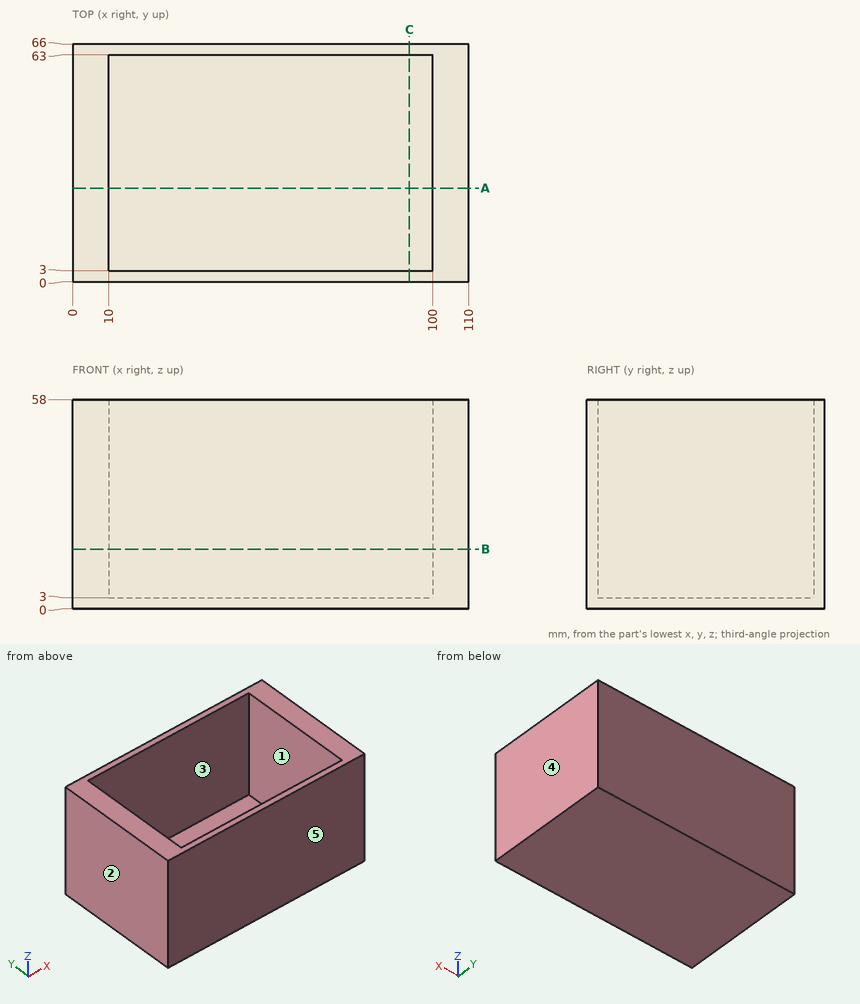
Part print with two shaded views. Sizes in mm from the minimum x, y, z corner. A direction names the side the tool comes from. Coordinates: 2 decimals unless noted, no trailing zeros. Write each loop counter-clockwise with the first axis right and the second up, starting at its lowest first coordinate (ties: lowest second). Pieces come first, ordered by that corner, then holes. Notation, with made-up numbers: (61, 62) -> (105, 62) arc R11 cw to (105, 69) -> close; hole circle Ø10 at (52.25, 76.25). An arc over 180 degrees is marked (long way). Return JSON: item names as keys, results as strings. Group by question number.
Q1. Cut at B-B, the plane z = 16.5. Give the cut face in (x, y).
Q2. Drill centre lines: line 1 (Y direction, x = 73, z = 9.5); line 2 (X direction, y = 10.5, z = 44); line 3 (Z direction, x = 31, y = 33.5). Where is each one in solid material? Low to high.
Q3. Which spindle directions (+Z, -Z, +X, -X, +Y, -Y) get a long thin tool onto all of the face, cutting with end or side? Do the marked faces 1 and 2. Say none if no direction does.
Q4. Pull direction Y, two halves, no side cores. Call the marked faces 3, 4 and 5: released by +Y, released by -Y, zero draft, split by the parting line, or undercut.
Q5. Cut at A-A, the plane y = 26. Give the cut face in (x, z).
Q6. Cut at C-C, the plane x = 93.5. Give the cut face in (y, z).
Q7. Flat gauge pins, fed straight in: pin 1 (6 mm diameter, centred on x = 92.5, y = 31, fed in from -Z); pin 2 (4 mm diameter, centred on x = 89.5, y = 57.5, fed in from +Z). Where does each tip first touch, or does it go through?
Returned:
{
 "1": {"outline": "(0, 0) -> (110, 0) -> (110, 66) -> (0, 66) -> close; hole (10, 3) -> (100, 3) -> (100, 63) -> (10, 63) -> close"},
 "2": {"line 1": "y = 0 to 3, 63 to 66", "line 2": "x = 0 to 10, 100 to 110", "line 3": "z = 0 to 3"},
 "3": {"face 1": "+Z", "face 2": "+Z, -Z, -X, +Y, -Y"},
 "4": {"face 3": "undercut", "face 4": "zero draft", "face 5": "released by -Y"},
 "5": {"outline": "(0, 0) -> (110, 0) -> (110, 58) -> (100, 58) -> (100, 3) -> (10, 3) -> (10, 58) -> (0, 58) -> close"},
 "6": {"outline": "(0, 0) -> (66, 0) -> (66, 58) -> (63, 58) -> (63, 3) -> (3, 3) -> (3, 58) -> (0, 58) -> close"},
 "7": {"pin 1": "stops at z = 0", "pin 2": "stops at z = 3"}
}
